Work out the finished part from the listing and answer in its coordinate system (mm). Face numbers are marked on the shaded views. A direction names the side the tool comes from. Round coordinates to 2 decimals unless told otherwise and drop trailing zeros. Loops run counter-clockwise (first coordinate to the right, second up) from the corner with the lowest first, then second, coordinate; pieces in that order, holes last. Notation, with made-up numbers: (62, -29) - (74, -29) arc R10 cw to (74, -21) - close; hole circle Ø8 at (57, -13.5). An arc over 180 degrees is marked (long way). Return JSON: item names as keys, results as strings.
from build123d import *

# Parameters (mm, degrees)
F2_W          = 230.1748
F2_H          = 279.4
F2_W_2        = 26.9748
F2_H_2        = 76.2
F3_DEPTH      = 21.972
F3_DEPTH_BACK = 79.63
F4_R          = 14.2875
F5_DEPTH      = 13.4884001
F5_DEPTH_BACK = 13.4884001
F6_SIZE       = 0.508
F7_SCALE      = 0.832549


with BuildPart() as f1:
    # F0 (on Front) → F1 (revolve)
    with BuildSketch(Plane.XZ):
        with BuildLine():
            ThreePointArc((29.972, 10.9855), (21.5151525193, 12.5638689957), (14.0702344541, 16.8746360971))
            ThreePointArc((14.0702344541, 16.8746360971), (-9.3163222306, 19.8980145013), (-21.971, 0))
            Line((-21.971, 0), (79.629, 0))
            Line((79.629, 0), (79.629, 8.17626))
            Line((79.629, 8.17626), (78.359, 9.44626))
            Line((78.359, 9.44626), (34.0925209982, 9.44626))
            Line((34.0925209982, 9.44626), (33.2232, 8.255))
            Line((33.2232, 8.255), (31.623, 8.255))
            ThreePointArc((31.623, 8.255), (30.7249743879, 8.6269743879), (30.353, 9.525))
            Line((30.353, 9.525), (30.353, 10.6045))
            Line((30.353, 10.6045), (29.972, 10.9855))
        make_face()
    revolve(axis=Axis((28.829, 0, 0), (1, 0, 0)))

    # F2 (on Right) → F3 (cut, two sides)
    with BuildSketch(Plane.YZ) as f3_sk:
        Rectangle(F2_W, F2_H)
        Rectangle(F2_W_2, F2_H_2, mode=Mode.SUBTRACT)
    extrude(amount=-F3_DEPTH, mode=Mode.SUBTRACT)
    extrude(f3_sk.sketch, amount=F3_DEPTH_BACK, mode=Mode.SUBTRACT)

    # F4 (on Front) → F5 (cut, two sides)
    with BuildSketch(Plane.XZ) as f5_sk:
        Circle(F4_R)
    extrude(amount=-F5_DEPTH, mode=Mode.SUBTRACT)
    extrude(f5_sk.sketch, amount=F5_DEPTH_BACK, mode=Mode.SUBTRACT)

    # F6
    f6_edges = [f1.edges().sort_by_distance(p)[0] for p in [
        (-14.2875, 13.4874, 0),
        (-14.2875, -13.4874, 0),
    ]]
    chamfer(f6_edges, length=F6_SIZE)


with BuildPart() as f1_1:
    # F7: moved
    add(f1.part.scale(F7_SCALE))


solid = f1_1.part
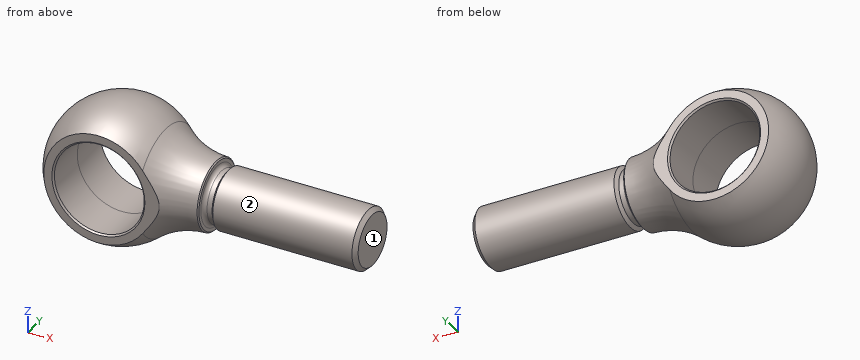
1) Flat-ended cylindrical pins translate along their axes: pin 1 (5 mm diameter, centred on y = -4, z = -11, fed in from -X); pin 2 (1.5 mm diameter, centred on x = 51, z = -7, fed in from -Y); pin 3 (5 mm diameter, centred on x = 50, y = 3.5, fed in from +Z). Find the tip coordinate at first contact, or state that the pin passes through.
Verdict:
{"pin 1": "stops at x = -15.81", "pin 2": "stops at y = -4.77", "pin 3": "stops at z = 7.8"}
2) Find the intervals of material crossed by L1, parallel to X at y = -0.25, z = -7; L2, parallel to X at y = 2.75, z = -0.5; L3, parallel to X at y = -7.75, z = 0, in increasing order.
Verdict:
{"L1": "x = -16.9 to -9.62, 9.62 to 25.82, 27.76 to 66.1", "L2": "x = -18.08 to -11.88, 11.88 to 66.3", "L3": "x = -16.57 to -11.9, 11.9 to 25.29, 28.3 to 65.35"}
3) Section A-A (x = 0) is taken. Give the vertices of the cut face in (y, z).
Verdict:
{"outline": "(-11.23, -14.44) arc R18.29 ccw to (11.23, -14.44) - (11.23, -12.32) - (10.81, -11.9) - (-10.81, -11.9) - (-11.23, -12.32) - close; (-11.23, 12.32) - (-10.81, 11.9) - (10.81, 11.9) - (11.23, 12.32) - (11.23, 14.44) arc R18.29 ccw to (-11.23, 14.44) - close"}
4) Section B-B (z = 0) is taken. Give the vertices of the cut face in (x, y).
Verdict:
{"outline": "(-14.44, -11.23) - (-12.32, -11.23) - (-11.9, -10.81) - (-11.9, 10.81) - (-12.32, 11.23) - (-14.44, 11.23) arc R18.29 ccw to start; (11.9, -10.81) - (12.32, -11.23) - (16.1, -11.23) arc R21.15 cw to (24.95, -9.15) - (25.27, -8.83) - (25.27, -7.93) arc R1.06 cw to (26.33, -6.87) - (27.66, -6.87) - (28.38, -7.86) - (65.24, -7.86) - (66.3, -6.81) - (66.3, 6.81) - (65.24, 7.86) - (28.38, 7.86) - (27.66, 6.87) - (26.33, 6.87) arc R1.06 cw to (25.27, 7.93) - (25.27, 8.83) - (24.95, 9.15) arc R21.15 cw to (16.1, 11.23) - (12.32, 11.23) - (11.9, 10.81) - close"}
5) A tool of negligible diameter and unlimited length cuts with its end or side. For the marked faces 1 and 2, from which of +Z, -Z, +X, -X, +Y, -Y can it reach the whole face along a straight path? Write none if from no direction.
Verdict:
{"face 1": "+Z, -Z, +X, +Y, -Y", "face 2": "+X"}
6) Section C-C (x = 34) is taken. Give the vertices of the cut face in (y, z), and give its area (3 significant figures).
Verdict:
{"outline": "circle Ø15.73 at (0, 0)", "area": "194 mm2"}
